Design review of the part built by this model. Coordinates are the model's own, in mm. Face numbers are marked on the shaded views. Give positions to 0.01 mm unless a question says otherwise; leave off trailing zeros. Loops run counter-clockwise (first coordinate to the right, second up) from the corner with the lowest first, then second, coordinate; pieces in that order, holes last.
from build123d import *

# Parameters (mm, degrees)
F0_R     = 23.9903837703
F1_DEPTH = 55.118
F2_R     = 5.08
F3_T     = -2.54
F5_DEPTH = 2.54
F7_DEPTH = 4.1402


# Not quite as in the source:
# - a shell that OpenCascade refuses in one call is made with other operations: the cavity is built on its own and cut out


with BuildPart() as f1:
    # F0 (on Top) → F1 (new body)
    with BuildSketch(Plane.XY):
        Circle(F0_R)
    extrude(amount=F1_DEPTH)

    # F2
    f2_edges = [f1.edges().sort_by_distance(p)[0] for p in [
        (-23.990384, 0, 55.118),
    ]]
    fillet(f2_edges, radius=F2_R)

    # F3: a shell. OpenCascade refuses it in one call, so the cavity is built on its own and cut out:
    # the body offset inwards by the wall thickness, plus a prism from it out through each open face.
    f3_core = offset(f1.part, amount=F3_T, mode=Mode.PRIVATE)
    f3_exits = [f3_core.faces().sort_by_distance(p)[0] for p in [
        (0, 0, 52.578),
    ]]
    add(f3_core, mode=Mode.SUBTRACT)
    extrude(f3_exits, amount=-F3_T, mode=Mode.SUBTRACT)

    # F4 (on Front) → F5 (join)
    with BuildSketch(Plane.XZ):
        with BuildLine():
            ThreePointArc((23.9537265152, 16.7385414243), (42.7735621339, 28.3666290343), (23.9537265152, 39.9947166443))
            Line((23.9537265152, 39.9947166443), (23.9537265152, 16.7385414243))
        make_face()
    extrude(amount=F5_DEPTH)

    # F6 (on Front) → F7 (cut)
    with BuildSketch(Plane.XZ):
        with BuildLine():
            ThreePointArc((23.9792838693, 21.4542429894), (37.798657028, 28.5622673109), (23.9792838693, 35.6702916324))
            Line((23.9792838693, 35.6702916324), (23.9792838693, 21.4542429894))
        make_face()
    extrude(amount=F7_DEPTH, mode=Mode.SUBTRACT)


solid = f1.part
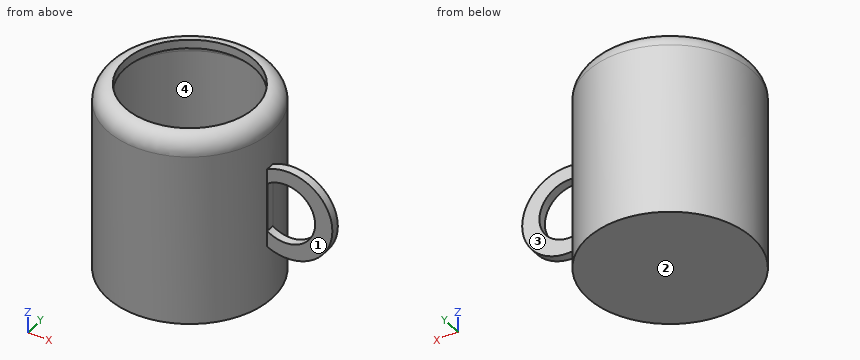
Q1. Take a section at C-C (x = 0). Give the boundary of the cut face in (y, z), plus the area to 3 significant figures.
Results:
outline: (-23.99, 0) - (23.99, 0) - (23.99, 50.04) arc R5.08 ccw to (18.91, 55.12) - (18.91, 52.58) arc R2.54 cw to (21.45, 50.04) - (21.45, 2.54) - (-21.45, 2.54) - (-21.45, 50.04) arc R2.54 cw to (-18.91, 52.58) - (-18.91, 55.12) arc R5.08 ccw to (-23.99, 50.04) - close
area: 394 mm2
Q2. Wall thickness on line 1 (Y direction, x = 0, z = 18); line 2 (Z direction, x = 1, y = -9); line 3 (X direction, y = 17.5, z = 31.5): over which ranges is each line inside the solid? List them lowest first.
Results:
line 1: y = -23.99 to -21.45, 21.45 to 23.99
line 2: z = 0 to 2.54
line 3: x = -16.41 to -12.4, 12.4 to 16.41
Q3. Draft analysis for pull direction Y (two halves, no side actions). For the marked faces 1, 2, 3 and 4, state which applies: pulls with the +Y half, pulls with the -Y half, needs draft (parallel to the pull), parting line crosses it, or undercut.
Results:
face 1: pulls with the -Y half
face 2: needs draft
face 3: pulls with the +Y half
face 4: undercut
Q4. Insertion check: pin 1 (5 mm diameter, centred on x = 30, y = 2, fed in from +Z); pin 2 (0.8 mm diameter, centred on y = -0.5, z = 30.5, fed in from +X); pin 3 (0.6 mm diameter, centred on y = -2, z = 31, fed in from -X). Each pin has a flat end and moves straight along its axis. Give the tip position at first contact, or say it passes through.
Results:
pin 1: stops at z = 41.37
pin 2: stops at x = 42.66
pin 3: stops at x = -23.93
Q5. Take a section at A-A (z = 28). Give the number of separate pieces and of enclosed holes in the cut face, plus the area to 3 significant figures.
Results:
separate pieces: 2
enclosed holes: 1
area: 375 mm2
Q6. Take a section at B-B (x = 36). Give the boundary of the cut face in (y, z), plus the area to 3 significant figures.
Results:
outline: (-2.54, 16.95) - (0, 16.95) - (0, 23.25) - (-2.54, 23.25) - close; (-2.54, 33.87) - (0, 33.87) - (0, 39.78) - (-2.54, 39.78) - close
area: 31.0 mm2
